Design review of the part built by this model. Coordinates are the model's own, in mm. A direction names the side the tool comes from. Coordinates: 2 decimals unless noted, no trailing zeros. Loops run counter-clockwise (first coordinate to the right, second up) from the corner with the lowest first, then second, coordinate; pieces in that order, holes last. Notation, with made-up numbers: (1, 80) -> (5, 80) arc R28 ccw to (5, 115) -> close; hole circle Ø9 at (-15.75, -11.75). An arc over 180 degrees is marked (long way). Answer in a Markdown table with one row per item.
```python
from build123d import *

# Parameters (mm, degrees)
SKETCH1_W           = 4
SKETCH1_H           = 17
BOSS_EXTRUDE1_DEPTH = 6
SKETCH2_W           = 2.8
SKETCH2_H           = 6.5
SKETCH2_W_2         = 1.5
SKETCH2_H_2         = 2.75
CUT_EXTRUDE1_DEPTH  = 19.466185313
CUT_EXTRUDE2_DEPTH  = 19.466185313
SKETCH4_W           = 2
SKETCH4_H           = 2.75
BOSS_EXTRUDE2_DEPTH = 2
SKETCH6_W           = 1.5
SKETCH6_H           = 1.7
SKETCH6_H_2         = 0.75
CUT_EXTRUDE3_DEPTH  = 2
BOSS_EXTRUDE3_REACH = 20.244
SKETCH7_W           = 2.6
SKETCH7_H           = 6.5
CUT_EXTRUDE4_DEPTH  = 10
SKETCH9_W           = 1.5
SKETCH9_H           = 17
CUT_EXTRUDE5_DEPTH  = 19.466185313


with BuildPart() as part:
    # Sketch1 → Boss-Extrude1 (new body)
    with BuildSketch(Plane.XY):
        with Locations((2, 8.5)):
            Rectangle(SKETCH1_W, SKETCH1_H)
    extrude(amount=BOSS_EXTRUDE1_DEPTH)

    # Sketch2 → Cut-Extrude1 (cut, through all)
    with BuildSketch(Plane.XY.offset(6)):
        with Locations((2.6, 9.25)):
            Rectangle(SKETCH2_W, SKETCH2_H)
        with Locations((3.25, 3.875)):
            Rectangle(SKETCH2_W_2, SKETCH2_H_2)
    extrude(amount=-CUT_EXTRUDE1_DEPTH, mode=Mode.SUBTRACT)

    # Sketch3 → Cut-Extrude2 (cut, through all)
    with BuildSketch(Plane.ZY):
        Polygon((0, 15.25), (0.75, 14.25), (0.75, 15.25), (2, 15.25), (2, 1.75), (0.75, 1.75), (0.75, 2.75), (0, 1.75), align=None)
    extrude(amount=-CUT_EXTRUDE2_DEPTH, mode=Mode.SUBTRACT)

    # Sketch4 → Boss-Extrude2 (add)
    with BuildSketch(Plane(origin=(4, 0, 0), x_dir=(0, 0, -1), z_dir=(1, 0, 0))):
        with Locations((-5, 3.875)):
            Rectangle(SKETCH4_W, SKETCH4_H)
    extrude(amount=-BOSS_EXTRUDE2_DEPTH)

    # Sketch6 → Cut-Extrude3 (cut)
    with BuildSketch(Plane(origin=(0, 0, 2), x_dir=(-1, 0, 0), z_dir=(0, 0, -1))):
        with Locations((-3.25, 13.35)):
            Rectangle(SKETCH6_W, SKETCH6_H)
        with Locations((-3.25, 5.625)):
            Rectangle(SKETCH6_W, SKETCH6_H_2)
    extrude(amount=-CUT_EXTRUDE3_DEPTH, mode=Mode.SUBTRACT)

    # Boss-Extrude3: up to this face of the body (flat: up to its plane)
    boss_extrude3_end = Plane(part.part.faces().sort_by_distance((4, 15.271515562, 3.544654939))[0])
    # Sketch7 → Boss-Extrude3 (add, up to the picked face)
    with BuildSketch(Plane(origin=(1.2, 0, 0), x_dir=(0, 0, -1), z_dir=(1, 0, 0)), mode=Mode.PRIVATE) as boss_extrude3_sk1:
        with Locations((-4.7, 9.25)):
            Rectangle(SKETCH7_W, SKETCH7_H)
    boss_extrude3_tool1 = split(extrude(boss_extrude3_sk1.sketch, amount=BOSS_EXTRUDE3_REACH, mode=Mode.PRIVATE), bisect_by=boss_extrude3_end, keep=Keep.BOTH, mode=Mode.PRIVATE)
    add(boss_extrude3_tool1.solids().sort_by(Axis((1.2, 9.25, 4.7), (1, 0, 0)))[0])

    # Sketch8 → Cut-Extrude4 (cut)
    with BuildSketch(Plane(origin=(0, 0, 3.4), x_dir=(-1, 0, 0), z_dir=(0, 0, -1))):
        with BuildLine():
            Line((-2.7, 10), (-4, 10))
            Line((-4, 10), (-4, 8))
            Line((-4, 8), (-2.7, 8))
            ThreePointArc((-2.7, 8), (-1.7, 9), (-2.7, 10))
        make_face()
    extrude(amount=-CUT_EXTRUDE4_DEPTH, mode=Mode.SUBTRACT)

    # Sketch9 → Cut-Extrude5 (cut, through all)
    with BuildSketch(Plane(origin=(4, 0, 0), x_dir=(0, 0, -1), z_dir=(1, 0, 0))):
        with Locations((-5.25, 8.5)):
            Rectangle(SKETCH9_W, SKETCH9_H)
    extrude(amount=-CUT_EXTRUDE5_DEPTH, mode=Mode.SUBTRACT)


solid = part.part
```
(1) Take a section at C-C on y = 10.25. Give the boundary of the cut face in (x, z), and give its area (3 significant figures).
Evaluation:
| item | result |
|---|---|
| outline | (0, 2) -> (1.2, 2) -> (1.2, 3.4) -> (4, 3.4) -> (4, 4.5) -> (0, 4.5) -> close |
| area | 6.08 mm² |
(2) To check wall thickness, follow probe 1 along Y at (x, z) = (2.8, 3.9); probe 2 along Y at (x, z) = (0.55, 1.3); probe 3 along Y at (x, z) = (2.15, 2.6). State the ranges of each line that lie inside material, in increasing order.
Evaluation:
| item | result |
|---|---|
| probe 1 | y = 0 to 2.5, 6 to 8, 10 to 12.5, 14.2 to 17 |
| probe 2 | y = 0 to 1.75, 15.25 to 17 |
| probe 3 | y = 0 to 6, 12.5 to 17 |
(3) Take a section at B-B on z = 4.15. Give the boundary of the cut face in (x, y).
Evaluation:
| item | result |
|---|---|
| outline | (0, 0) -> (4, 0) -> (4, 8) -> (2.7, 8) arc R1 cw to (2.7, 10) -> (4, 10) -> (4, 17) -> (0, 17) -> close |
(4) Tool access review of faces 1 (the flat face through (4, 2, 3)), 2 (the flat face through (3, 8, 4)), 3 (the flat face through (2, 15, 0.75)), 4 (the flat face through (0, 8, 3)), 5 (the flat face through (2, 10, 3.4)): name each direction out of +Z, -Z, +X, -X, +Y, -Y from which nothing blocks a thin tool from reaching the whole face with its end or side.
Evaluation:
| item | result |
|---|---|
| face 1 | +Z, -Z, +X, +Y, -Y |
| face 2 | +Z, -Z, +X |
| face 3 | +X, -X |
| face 4 | +Z, -Z, -X, +Y, -Y |
| face 5 | -Z, +X |
(5) Take a section at D-D on x = 1.55. Give the boundary of the cut face in (y, z).
Evaluation:
| item | result |
|---|---|
| outline | (0, 0) -> (1.75, 0) -> (2.75, 0.75) -> (1.75, 0.75) -> (1.75, 2) -> (6, 2) -> (6, 3.4) -> (12.5, 3.4) -> (12.5, 2) -> (15.25, 2) -> (15.25, 0.75) -> (14.25, 0.75) -> (15.25, 0) -> (17, 0) -> (17, 4.5) -> (0, 4.5) -> close |
(6) Take a section at A-A on x = 3.15. Give the boundary of the cut face in (y, z), and give its area (3 significant figures).
Evaluation:
| item | result |
|---|---|
| outline | (0, 0) -> (1.75, 0) -> (2.5, 0.56) -> (2.5, 0.75) -> (1.75, 0.75) -> (1.75, 2) -> (2.5, 2) -> (2.5, 4) -> (6, 4) -> (6, 3.4) -> (8, 3.4) -> (8, 4.5) -> (0, 4.5) -> close; (10, 3.4) -> (12.5, 3.4) -> (12.5, 4) -> (14.2, 4) -> (14.2, 2) -> (15.25, 2) -> (15.25, 0.75) -> (14.25, 0.75) -> (15.25, 0) -> (17, 0) -> (17, 4.5) -> (10, 4.5) -> close |
| area | 28.5 mm² |
(7) For pin 1 (1.1 mm diameter, centred on y = 9, z = 3, fed in from +X); pin 2 (1.6 mm diameter, centred on x = 3.5, y = 5, fed in from -Z), all flat-tipped, find the tip position at first contact; note any pin that passes through.
Evaluation:
| item | result |
|---|---|
| pin 1 | stops at x = 1.77 |
| pin 2 | stops at z = 4 |
(8) Draft analysis for pull direction Z (two halves, no side actions). For faces 6 (the flat face through (1.972, 14.757, 0.37)), 7 (the flat face through (1, 9, 2)), 8 (the flat face through (1.2, 9, 3)), state which applies: pulls with the +Z half, pulls with the -Z half, needs draft (parallel to the pull), parting line crosses it, or undercut.
Evaluation:
| item | result |
|---|---|
| face 6 | pulls with the -Z half |
| face 7 | undercut |
| face 8 | needs draft |
